Source: CAD feature listing. Evaluate the final solid. Frame: model axes, mm. A direction names the side the tool comes from. Round coordinates to 2 decimals unless told otherwise and drop trailing zeros. Loops run counter-clockwise (first coordinate to the right, second up) from the corner with the lowest first, then second, coordinate; pieces in that order, holes last.
Item 1: Section query D-D on y = -55. Return loops of the section in (x, z), then the cut area to 3 significant figures.
Item 2: Pull-direction query (Z, two-part tool) for faces 4 (the flat face through (55, 0, -70)), 5 (the flat face through (80.66, 1.25, -99.53)), 6 (the flat face through (103.473, -9.53, -25.673)); classes: released by +Z, released by -Z, zero draft, split by the parting line, or undercut.
Item 3: Section query A-A on y = -32. Return loops of the section in (x, z), then the cut area to 3 significant figures.
Item 4: Section query C-C on y = -41. Return loops of the section in (x, z).
Item 5: Section query B-B on x = 15.5. Return loops of the section in (y, z).
Item 6: Ray query, L1, parallel to Y at x = 52, z = -23; L2, parallel to Z at x = 109, y = -26; L3, parallel to Z at x = 90.5, y = -46.5. Return the intervals inside material, ascending.
Item 7: Access query for faces 1 (the cylindrical face through (108.42, 1.25, -19.68)), 2 (the flat face through (68.11, 1.25, -119.5)), 3 (the flat face through (114.65, 1.25, -1)). Directions: +Z, -Z, +X, -X, +Y, -Y. A direction counts if a zero-diameter tool reaches every point of the face in a straight line with its end or side. Return the directions, or none.
Item 8: First-contact query: P1, Ø2, axis at x = 68, y = -27, coming from the +Z side; P2, Ø6, axis at x = 107, y = -63.5, coming from the -Z side; P3, Ø4, axis at x = 71.41, z = -115.88, coming from the -Y side. Flat tips, straight axial feed; report the tip coordinate or a pass-through.
```python
from build123d import *

# Parameters (mm, degrees)
SKETCH3_R               = 3.175
BOSS_EXTRUDE1_DEPTH     = 2.54
BOSS_EXTRUDE2_DEPTH     = 76.2
CUT_EXTRUDE1_DEPTH      = 159.608869597
CUT_EXTRUDE1_DEPTH_BACK = 159.608869597


with BuildPart() as part:
    # Sketch3 → Boss-Extrude1 (new body)
    with BuildSketch(Plane(origin=(0, 0, 0), x_dir=(1, 0, 0), z_dir=(0, 1, 0))):
        with BuildLine():
            Line((-0.667272367, 91.211244064), (42.072585982, 45.579833776))
            Line((42.072585982, 45.579833776), (62.900199296, -34.141504839))
            Line((62.900199296, -34.141504839), (98.113451188, -35.418279698))
            Line((98.113451188, -35.418279698), (119.317385982, -15.557986891))
            Line((119.317385982, -15.557986891), (109.850299083, 18.019409705))
            ThreePointArc((109.850299083, 18.019409705), (114.061816463, 23.863253473), (107.41792498, 26.646434133))
            Line((107.41792498, 26.646434133), (89.543483254, 90.042621912))
            Line((89.543483254, 90.042621912), (71.515910096, 109.289844975))
            Line((71.515910096, 109.289844975), (77.978605526, 115.34301505))
            Line((77.978605526, 115.34301505), (71.293896806, 122.479975678))
            Line((71.293896806, 122.479975678), (64.831201375, 116.426805602))
            Line((64.831201375, 116.426805602), (46.803628217, 135.674028665))
            Line((46.803628217, 135.674028665), (-0.667272367, 91.211244064))
        make_face()
        with Locations(Location((71.405004975, 115.88499878, 0), (0, 0, 270))):
            Circle(SKETCH3_R, mode=Mode.SUBTRACT)
        with Locations(Location((109.633944273, 22.61482283, 0), (0, 0, 270))):
            Circle(SKETCH3_R, mode=Mode.SUBTRACT)
    extrude(amount=BOSS_EXTRUDE1_DEPTH)

    # Sketch4 → Boss-Extrude2 (add)
    with BuildSketch(Plane(origin=(0, 2.54, 0), x_dir=(1, 0, 0), z_dir=(0, 1, 0))):
        with BuildLine():
            Line((46.803628217, 129.736619854), (5.454929405, 91.008087929))
            Line((5.454929405, 91.008087929), (46.353114934, 47.342948269))
            Line((46.353114934, 47.342948269), (61.1366863, -10.500532511))
            ThreePointArc((61.1366863, -10.500532511), (94.212402493, -28.283463558), (108.844487247, 6.301760657))
            Line((108.844487247, 6.301760657), (86.410796294, 87.200194916))
            Line((86.410796294, 87.200194916), (46.803628217, 129.736619854))
        make_face()
    extrude(amount=-BOSS_EXTRUDE2_DEPTH)

    # Sketch14 → Cut-Extrude1 (cut, two sides: drawn at the far end of the back side and taken through both)
    with BuildSketch(Plane(origin=(50.531559178, 0, -13.201631997), x_dir=(0.25277120811930814, 0, 0.9675260804473983), z_dir=(-0.9675260804473983, 0, 0.25277120811930814)).offset(-CUT_EXTRUDE1_DEPTH_BACK)):
        with BuildLine():
            Line((-119.586340422, -76.2), (-7.964682874, -76.2))
            Line((-7.964682874, -76.2), (52.762632555, -76.2))
            ThreePointArc((52.762632555, -76.2), (9.204123856, -25.310156709), (-52.816161516, 0))
            Line((-52.816161516, 0), (-119.586340422, 0))
            Line((-119.586340422, 0), (-119.586340422, -76.2))
        make_face()
    extrude(amount=CUT_EXTRUDE1_DEPTH + CUT_EXTRUDE1_DEPTH_BACK, mode=Mode.SUBTRACT)


solid = part.part
```
Data:
1. outline: (68.51, 22.95) - (109.95, 12.13) arc R25.4 ccw to start
1. area: 355 mm2
2. face 4: zero draft
2. face 5: undercut
2. face 6: released by -Z
3. outline: (59.19, 2.9) - (107.87, -9.82) - (108.84, -6.3) arc R25.4 ccw (long way) to (61.14, 10.5) - close
3. area: 1,420 mm2
4. outline: (61.65, 12.28) - (110.7, -0.54) arc R25.4 ccw to start
5. outline: (0, -106.35) - (2.54, -106.35) - (2.54, -73.95) - (0, -73.95) - close
6. L1: y = 0 to 2.54
6. L2: z = -5.96 to 14.61
6. L3: z = 10.03 to 29.28
7. face 1: +Y, -Y
7. face 2: -Z, +Y, -Y
7. face 3: +X, +Y, -Y
8. P1: stops at z = 23.4
8. P2: stops at z = 16.84
8. P3: passes through
